from build123d import *

# Parameters (mm, degrees)
ARRAY_X_COUNT = 2
ARRAY_X_PITCH = 10
ARRAY_Y_COUNT = 6
ARRAY_Y_PITCH = 10
BOX_W         = 20
BOX_H         = 60
BOX_DEPTH     = 10
FILLET_R      = 2
FILLET001_R   = 1


with BuildPart() as obj1:
    # Cone → Cone (revolve)
    with BuildSketch(Plane(origin=(5, 5, 1), x_dir=(1, 0, 0), z_dir=(0, -1, 0))):
        Polygon((0, 0), (1, 0), (4, 10), (0, 10), align=None)
    revolve(axis=Axis((5, 5, 1), (0, 0, 1)))

    # Array X: obj1_2


with BuildPart() as obj1_1:
    add(obj1.part)
    with Locations(*[(i * ARRAY_X_PITCH, 0, 0) for i in range(1, ARRAY_X_COUNT)]):
        add(obj1.part)

    # Array Y: obj1 ×6


with BuildPart() as obj1_2:
    add(obj1_1.part)
    with Locations(*[(0, i * ARRAY_Y_PITCH, 0) for i in range(1, ARRAY_Y_COUNT)]):
        add(obj1_1.part)


with BuildPart() as fillet001:
    # Box → Box (new body)
    with BuildSketch(Plane.XY):
        with Locations((10, 30)):
            Rectangle(BOX_W, BOX_H)
    extrude(amount=BOX_DEPTH)

    # Fillet
    fillet_edges = [fillet001.edges().sort_by_distance(p)[0] for p in [
        (0, 0, 5),
        (0, 60, 5),
        (20, 0, 5),
        (20, 60, 5),
    ]]
    fillet(fillet_edges, radius=FILLET_R)

    # Cut: cut obj1
    add(obj1_2.part, mode=Mode.SUBTRACT)

    # Fillet001
    fillet001_edges = [fillet001.edges().sort_by_distance(p)[0] for p in [
        (0, 30, 10),
        (0.585786, 0.585786, 10),
        (0.585786, 59.414214, 10),
        (10, 0, 10),
        (10, 60, 10),
        (19.414214, 0.585786, 10),
        (19.414214, 59.414214, 10),
        (20, 30, 10),
    ]]
    fillet(fillet001_edges, radius=FILLET001_R)


solid = fillet001.part
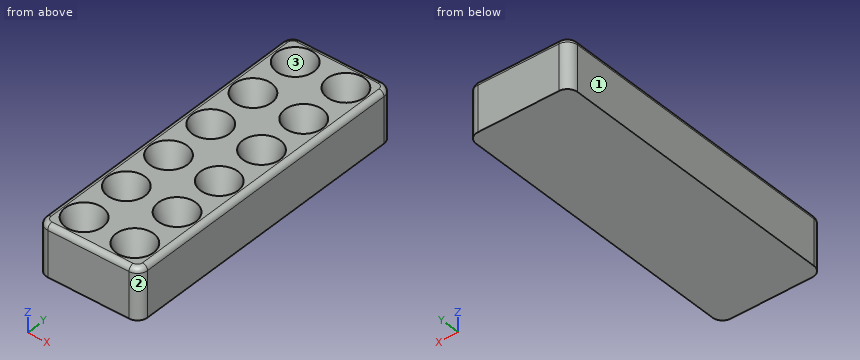
The model under review builds one solid part; all positions refer to its coordinate system, in mm. Face numbers are marked on the shaded views. Round coordinates to 2 decimals unless told otherwise and drop trailing zeros. Loops run counter-clockwise (first coordinate to the right, second up) from the corner with the lowest first, then second, coordinate; pieces in that order, holes last. Notation, with made-up numbers: (24, -28) -> (44, -28) arc R13 cw to (44, -12) -> close; hole circle Ø6 at (29.5, -1). An arc over 180 degrees is marked (long way). One line per question, with ' | ' between items. Start each with the question number.
Item 1: Draft analysis for pull direction X (two halves, no side actions). For the marked faces 1, 2 and 3, state which applies: +X half, -X half, draft (parallel to the pull), parting line (faces both ways), or undercut.
Item 2: Add section A-A, the plane z = 2. Count the separate pieces of the cut face and the enclosed holes in it, then the cut area to 3 significant figures.
Item 3: Add section B-B, the plane y = 15. Write out the cut boundary in (x, z), then the cut area to 3 significant figures.
Item 4: Wall thickness on line 1 along X through (y, z) = (55, 1.5); line 2 along X through (y, z) = (5, 7.5); line 3 along Y through (x, z) = (18.5, 2.5): over which ranges is each line inside the solid? List them lowest first. Write a range as [from, to].
Item 5: For pin 1 (0.6 mm diameter, centred on x = 5, y = 55, fed in from +Z), flat-tipped, find the tip position at first contact; note if it passes through.
Return value:
1) face 1: -X half | face 2: +X half | face 3: undercut
2) separate pieces: 1 | enclosed holes: 12 | area: 1,130 mm2
3) outline: (0, 0) -> (20, 0) -> (20, 9) arc R1 ccw to (19, 10) -> (18.7, 10) -> (16, 1) -> (14, 1) -> (11.3, 10) -> (8.7, 10) -> (6, 1) -> (4, 1) -> (1.3, 10) -> (1, 10) arc R1 ccw to (0, 9) -> close | area: 115 mm2
4) line 1: x = [0, 3.85], [6.15, 13.85], [16.15, 20] | line 2: x = [0, 2.05], [7.95, 12.05], [17.95, 20] | line 3: y = [0.06, 59.94]
5) pin 1: stops at z = 1
